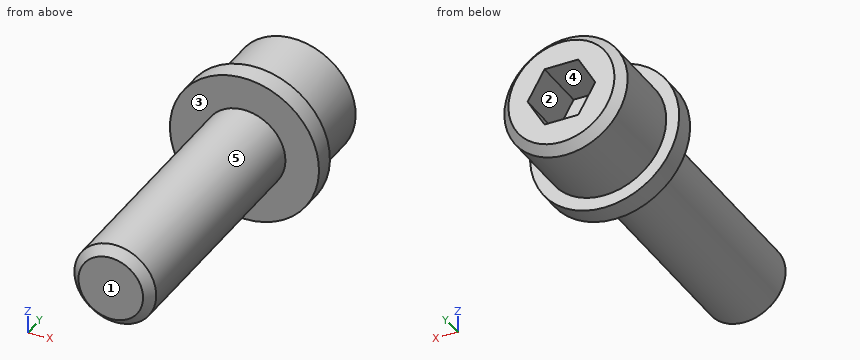
from build123d import *

# Parameters (mm, degrees)
CUT_EXTRUDE1_DEPTH = 6.4
CHAMFER1_SIZE      = 1


with BuildPart() as part:
    # Sketch1 → Revolve1 (revolve)
    with BuildSketch(Plane.XY, mode=Mode.PRIVATE) as revolve1_sk:
        Polygon((0, 0), (0, 41.3), (7.15, 41.3), (7.15, 31.8), (8.65, 31.8), (8.65, 29.4), (4.75, 29.4), (4.75, 0), align=None)
    revolve(revolve1_sk.sketch.rotate(Axis((0, 0, 0), (0, 1, 0)), 90), axis=Axis((0, 0, 0), (0, 1, 0)))

    # Sketch2 → Cut-Extrude1 (cut)
    with BuildSketch(Plane(origin=(0, 41.3, 0), x_dir=(1, 0, 0), z_dir=(0, 1, 0))):
        Polygon((3.92598183, 0), (1.962990915, 3.4), (-1.962990915, 3.4), (-3.92598183, 0), (-1.962990915, -3.4), (1.962990915, -3.4), align=None)
    extrude(amount=-CUT_EXTRUDE1_DEPTH, mode=Mode.SUBTRACT)

    # Chamfer1
    chamfer1_edges = [part.edges().sort_by_distance(p)[0] for p in [
        (0, 0, 4.75),
        (0, 41.3, 7.15),
    ]]
    chamfer(chamfer1_edges, length=CHAMFER1_SIZE)


solid = part.part
Here's how the part is built. I have some questions about the finished solid (model axes, mm). Face numbers are marked on the shaded views. A direction names the side the tool comes from. Give positions to 0.01 mm unless a question says otherwise; leave off trailing zeros. Loops run counter-clockwise (first coordinate to the right, second up) from the corner with the lowest first, then second, coordinate; pieces in that order, holes last. Notation, with made-up numbers: (71, 58) -> (110, 58) arc R11 cw to (110, 63) -> close; hole circle Ø7 at (-15.5, 80). An arc over 180 degrees is marked (long way). Answer as a JSON object with one key per item and string values. Group by question number.
Item 1: On a 3-axis mill with a long thin cutter (end or side, diameter ignored), from which of +Z, -Z, +X, -X, +Y, -Y can I reach the whole of each face in a straight line? I mean the marked faces 1 and 2. Say none if no direction works.
Item 2: Imagine slicing it at B-B on y = 3.5. Write out the boundary of the cut face in (x, z), then the cut area to 3 significant figures.
Item 3: Will these pins go through, and if not, where does the flat tip stop? pin 1 (3 mm diameter, centred on x = 1, y = 36.5, fed in from -Z); pin 2 (6 mm diameter, centred on x = -6.5, y = 28, fed in from -Z); pin 3 (2 mm diameter, centred on x = -5, y = 24.5, fed in from -Z).
Item 4: Imagine slicing it at C-C on y = 33. Write out the boundary of the cut face in (x, z).
Item 5: Imagine slicing it at A-A on x = 0. Write out the boundary of the cut face in (y, z), then the cut area to 3 significant figures.
Item 6: I need wall thicknesses on L1, parallel to Y at x = 6.75, z = -3.25; L2, parallel to Y at x = 3.25, z = 1; L3, parallel to Z at x = 3.5, y = 38. Which ranges of each line are inside material? Lowest first, please.
Item 7: Thinking about a two-plate mould opening in X: for the marked faces 3, 4 and 5, which applies, pulls with the +X half, pulls with the -X half, needs draft (parallel to the pull), parting line crosses it, or undercut?
Answer list:
{
 "1": {"face 1": "+Z, -Z, +X, -X, -Y", "face 2": "+Y"},
 "2": {"outline": "circle Ø9.5 at (0, 0)", "area": "70.9 mm2"},
 "3": {"pin 1": "stops at z = -7.15", "pin 2": "stops at z = -7.75", "pin 3": "stops at z = -2.56"},
 "4": {"outline": "circle Ø14.3 at (0, 0)"},
 "5": {"outline": "(0, -3.75) -> (1, -4.75) -> (29.4, -4.75) -> (29.4, -8.65) -> (31.8, -8.65) -> (31.8, -7.15) -> (40.3, -7.15) -> (41.3, -6.15) -> (41.3, -3.4) -> (34.9, -3.4) -> (34.9, 3.4) -> (41.3, 3.4) -> (41.3, 6.15) -> (40.3, 7.15) -> (31.8, 7.15) -> (31.8, 8.65) -> (29.4, 8.65) -> (29.4, 4.75) -> (1, 4.75) -> (0, 3.75) -> close", "area": "411 mm2"},
 "6": {"L1": "y = 29.4 to 31.8", "L2": "y = 0 to 34.9", "L3": "z = -6.23 to -0.74, 0.74 to 6.23"},
 "7": {"face 3": "needs draft", "face 4": "undercut", "face 5": "parting line crosses it"}
}
